```python
from build123d import *

# Parameters (mm, degrees)
SKETCH_1_R               = 85
SKETCH_1_R_2             = 3
EXTRUDE_1_DEPTH          = 6
SKETCH_2_R               = 1.55
CUT_EXTRUDE_1_DEPTH      = 121.357799913
PATTERN_CIRCULAR_2_COUNT = 4
CHAMFER_1_SIZE           = 3


with BuildPart() as part:
    # 草图1 → 凸台-拉伸1 (new body)
    with BuildSketch(Plane.XY):
        Circle(SKETCH_1_R)
        Circle(SKETCH_1_R_2, mode=Mode.SUBTRACT)
        with BuildLine():
            Line((-31.725622255, -22.214519858), (-52.610992631, -36.838613633))
            ThreePointArc((-52.610992631, -36.838613633), (-60.837871991, -38.331841306), (-67.323181147, -33.054338296))
            ThreePointArc((-67.323181147, -33.054338296), (-75, 0), (-67.323181147, 33.054338296))
            ThreePointArc((-67.323181147, 33.054338296), (-60.837871698, 38.331841382), (-52.610992136, 36.838613286))
            Line((-52.610992136, 36.838613286), (-31.725621944, 22.214519639))
            ThreePointArc((-31.725621944, 22.214519639), (-27.910605359, 16.986540764), (-28.096039964, 10.517249561))
            ThreePointArc((-28.096039964, 10.517249561), (-30, 0), (-28.096039964, -10.517249561))
            ThreePointArc((-28.096039964, -10.517249561), (-27.910605416, -16.986540946), (-31.725622255, -22.214519858))
        make_face(mode=Mode.SUBTRACT)
        with BuildLine():
            Line((22.214519858, -31.725622255), (36.838613633, -52.610992631))
            ThreePointArc((36.838613633, -52.610992631), (38.331841306, -60.837871991), (33.054338296, -67.323181147))
            ThreePointArc((33.054338296, -67.323181147), (0, -75), (-33.054338296, -67.323181147))
            ThreePointArc((-33.054338296, -67.323181147), (-38.331841382, -60.837871698), (-36.838613286, -52.610992136))
            Line((-36.838613286, -52.610992136), (-22.214519639, -31.725621944))
            ThreePointArc((-22.214519639, -31.725621944), (-16.986540764, -27.910605359), (-10.517249561, -28.096039964))
            ThreePointArc((-10.517249561, -28.096039964), (0, -30), (10.517249561, -28.096039964))
            ThreePointArc((10.517249561, -28.096039964), (16.986540946, -27.910605416), (22.214519858, -31.725622255))
        make_face(mode=Mode.SUBTRACT)
        with BuildLine():
            ThreePointArc((-10.517249561, 28.096039964), (-16.986540946, 27.910605416), (-22.214519858, 31.725622255))
            Line((-22.214519858, 31.725622255), (-36.838613633, 52.610992631))
            ThreePointArc((-36.838613633, 52.610992631), (-38.331841306, 60.837871991), (-33.054338296, 67.323181147))
            ThreePointArc((-33.054338296, 67.323181147), (0, 75), (33.054338296, 67.323181147))
            ThreePointArc((33.054338296, 67.323181147), (38.331841382, 60.837871698), (36.838613286, 52.610992136))
            Line((36.838613286, 52.610992136), (22.214519639, 31.725621944))
            ThreePointArc((22.214519639, 31.725621944), (16.986540764, 27.910605359), (10.517249561, 28.096039964))
            ThreePointArc((10.517249561, 28.096039964), (5.3440996, 29.520172755), (0, 30))
            ThreePointArc((0, 30), (-5.3440996, 29.520172755), (-10.517249561, 28.096039964))
        make_face(mode=Mode.SUBTRACT)
        with BuildLine():
            Line((31.725622255, 22.214519858), (52.610992631, 36.838613633))
            ThreePointArc((52.610992631, 36.838613633), (60.837871991, 38.331841306), (67.323181147, 33.054338296))
            ThreePointArc((67.323181147, 33.054338296), (75, 0), (67.323181147, -33.054338296))
            ThreePointArc((67.323181147, -33.054338296), (60.837871698, -38.331841382), (52.610992136, -36.838613286))
            Line((52.610992136, -36.838613286), (31.725621944, -22.214519639))
            ThreePointArc((31.725621944, -22.214519639), (27.910605359, -16.986540764), (28.096039964, -10.517249561))
            ThreePointArc((28.096039964, -10.517249561), (30, 0), (28.096039964, 10.517249561))
            ThreePointArc((28.096039964, 10.517249561), (27.910605416, 16.986540946), (31.725622255, 22.214519858))
        make_face(mode=Mode.SUBTRACT)
    extrude(amount=EXTRUDE_1_DEPTH)

    # 草图2 → 切除-拉伸1 (cut, through all)
    with BuildSketch(Plane.XY.offset(6)):
        with Locations((0, 10)):
            Circle(SKETCH_2_R)
    cut_extrude_1 = extrude(amount=-CUT_EXTRUDE_1_DEPTH, mode=Mode.SUBTRACT)

    # 阵列(圆周)2: 切除-拉伸1 ×4 about axis
    pattern_circular_2_axis = Axis((0, 0, 0), (0, 0, 1))
    for i in range(1, PATTERN_CIRCULAR_2_COUNT):
        add(cut_extrude_1.rotate(pattern_circular_2_axis, i * 360 / PATTERN_CIRCULAR_2_COUNT), mode=Mode.SUBTRACT)

    # 倒角1
    chamfer_1_edges = [part.edges().sort_by_distance(p)[0] for p in [
        (-85, 0, 0),
    ]]
    chamfer(chamfer_1_edges, length=CHAMFER_1_SIZE)


solid = part.part
```
The model under review builds one solid part; all positions refer to its coordinate system, in mm. A direction names the side the tool comes from. Give positions to 0.01 mm unless a question says otherwise; leave off trailing zeros. Write each question's results on one line, items separated by ' | '. Start each with the question number.
1. Mouldability with a two-part tool opening along X and no side actions: class faces 1 (the conical face through (-17.808, -80.192, 0.146)), 2 (the flat face through (0, -6, 0)), 3 (the cylindrical face through (-17.075, -27.938, 2.958)) as released by +X, released by -X, zero draft, split by the parting line, or undercut.
2. For probe 1 along Y at (x, z) = (0, 3.05); probe 2 along X at (y, z) = (17.5, 4); probe 3 along X at (y, z) = (-6, 1), list the stretches that pass through material, from the lowest coordinate up. Write a range as [from, to].
3. For faces 4 (the cylindrical face through (16.898, -27.884, 2.958)), 5 (the flat face through (-20, 1, 6)), list the 3-axis set-ups (+Z, -Z, +X, -X, +Y, -Y) from which the entire face can be reached by the end or side of a thin tool; tool diameter is ignored.
4. We need section A-A (z = 2). Count the separate pieces of the cut face and the enclosed holes in it, and give its area (3 significant figures).
5. Insertion check: pin 1 Ø4 at (x, y) = (0, -10) entering from +Z; pin 2 Ø3 at (x, z) = (15.5, 2.5) entering from -Y; pin 3 Ø1 at (x, z) = (6, 5.5) entering from -Y. Each pin has a flat end and moves straight along its axis. Give the tip position at first contact, or say it passes through.
Results found:
1) face 1: split by the parting line | face 2: zero draft | face 3: undercut
2) probe 1: y = [-85, -75], [-30, -11.55], [-8.45, -3], [3, 8.45], [11.55, 30], [75, 85] | probe 2: x = [-83.18, -72.93], [-28.09, 28.09], [72.93, 83.18] | probe 3: x = [-82.78, -74.76], [-29.39, 29.39], [74.76, 82.78]
3) face 4: +Z, -Z | face 5: +Z, +X, -X, +Y, -Y
4) separate pieces: 1 | enclosed holes: 9 | area: 10,900 mm^2
5) pin 1: stops at z = 6 | pin 2: stops at y = -83.82 | pin 3: stops at y = -84.82
